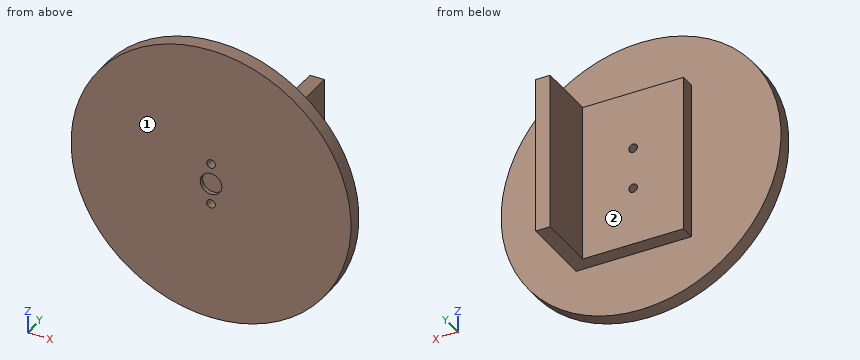
from build123d import *

# Parameters (mm, degrees)
SKETCH2_R           = 48.5
BOSS_EXTRUDE1_DEPTH = 5
SKETCH6_W           = 35
SKETCH6_H           = 55
BOSS_EXTRUDE2_DEPTH = 5
SKETCH4_R           = 1.5
CUT_EXTRUDE2_DEPTH  = 70.314500647
SKETCH5_R           = 3.75
CUT_EXTRUDE3_DEPTH  = 1.5
SKETCH7_W           = 5
SKETCH7_H           = 55
BOSS_EXTRUDE3_DEPTH = 25.5


with BuildPart() as part:
    # Sketch2 → Boss-Extrude1 (new body)
    with BuildSketch(Plane(origin=(0, 0, 0), x_dir=(1, 0, 0), z_dir=(0, 1, 0))):
        with Locations(Location((0, 0, 0), (0, 0, 270))):
            Circle(SKETCH2_R)
    extrude(amount=BOSS_EXTRUDE1_DEPTH)

    # Sketch6 → Boss-Extrude2 (add)
    with BuildSketch(Plane(origin=(0, 5, 0), x_dir=(1, 0, 0), z_dir=(0, 1, 0))):
        Rectangle(SKETCH6_W, SKETCH6_H)
    extrude(amount=BOSS_EXTRUDE2_DEPTH)

    # Sketch4 → Cut-Extrude2 (cut, through all)
    with BuildSketch(Plane.XZ):
        with Locations(Location((0, 7.25, 0), (0, 0, 270))):
            Circle(SKETCH4_R)
        with Locations(Location((0, -7.25, 0), (0, 0, 270))):
            Circle(SKETCH4_R)
    extrude(amount=-CUT_EXTRUDE2_DEPTH, mode=Mode.SUBTRACT)

    # Sketch5 → Cut-Extrude3 (cut)
    with BuildSketch(Plane.XZ):
        with Locations(Location((0, 0, 0), (0, 0, 270))):
            Circle(SKETCH5_R)
    extrude(amount=-CUT_EXTRUDE3_DEPTH, mode=Mode.SUBTRACT)

    # Sketch7 → Boss-Extrude3 (add)
    with BuildSketch(Plane(origin=(0, 5, 0), x_dir=(1, 0, 0), z_dir=(0, 1, 0))):
        with Locations((20, 0)):
            Rectangle(SKETCH7_W, SKETCH7_H)
    extrude(amount=BOSS_EXTRUDE3_DEPTH)


solid = part.part
The listing builds one solid part. Answer for the finished solid, in the listing's coordinates (mm). Face numbers are marked on the shaded views. A direction names the side the tool comes from. Give positions to 0.01 mm unless a question says otherwise; leave off trailing zeros. Write each loop counter-clockwise with the first axis right and the second up, starting at its lowest first coordinate (ties: lowest second). Pieces come first, ordered by that corner, then holes.
1) Section D-D (y = 15) is taken. Write down the section's boundary in (x, z).
2) Given P1, Ø8, axis at y = 25, z = 32.5, coming from the -X side; P2, Ø4, axis at y = 5.5, z = 6, coming from the +X side; P3, Ø2, axis at x = -2, z = 0, coming from the -Y side; P4, Ø6, axis at y = 24, z = 3, coming from the -X side, each flat-ended and moving along its own axis, determine where each tip first touches the part or whether it passes through.
3) Section B-B (y = 7) is taken. Write down the section's boundary in (x, z), and give its area (3 significant figures).
4) A tool of negligible diameter and unlimited length cuts with its end or side. For the marked faces 1 and 2, from which of +Z, -Z, +X, -X, +Y, -Y can it reach the whole face along a straight path? Write none if from no direction.
5) Section C-C (z = 0) is taken. Write down the section's boundary in (x, y), and give its area (3 significant figures).
6) Find the intervals of material crossed by L1, parallel to X at y = 6.5, z = -7.25; L2, parallel to Y at x = 35.5, z = -7; L3, parallel to X at y = 5.5, z = -16, in increasing order.
7) Section A-A (x = 0) is taken. Write down the section's boundary in (y, z).
Response:
1. outline: (17.5, -27.5) - (22.5, -27.5) - (22.5, 27.5) - (17.5, 27.5) - close
2. P1: passes through
2. P2: stops at x = 48.33
2. P3: stops at y = 1.5
2. P4: stops at x = 17.5
3. outline: (-17.5, -27.5) - (22.5, -27.5) - (22.5, 27.5) - (-17.5, 27.5) - close; hole circle Ø3 at (0, -7.25); hole circle Ø3 at (0, 7.25)
3. area: 2,190 mm2
4. face 1: +Z, -Z, +X, -X, -Y
4. face 2: +Z, -Z, -X, +Y
5. outline: (-48.5, 0) - (-3.75, 0) - (-3.75, 1.5) - (3.75, 1.5) - (3.75, 0) - (48.5, 0) - (48.5, 5) - (22.5, 5) - (22.5, 30.5) - (17.5, 30.5) - (17.5, 10) - (-17.5, 10) - (-17.5, 5) - (-48.5, 5) - close
5. area: 776 mm2
6. L1: x = -17.5 to -1.5, 1.5 to 22.5
6. L2: y = 0 to 5
6. L3: x = -17.5 to 22.5
7. outline: (0, -48.5) - (5, -48.5) - (5, -27.5) - (10, -27.5) - (10, -8.75) - (0, -8.75) - close; (0, -5.75) - (10, -5.75) - (10, 5.75) - (0, 5.75) - (0, 3.75) - (1.5, 3.75) - (1.5, -3.75) - (0, -3.75) - close; (0, 8.75) - (10, 8.75) - (10, 27.5) - (5, 27.5) - (5, 48.5) - (0, 48.5) - close
